Autodesk Inventor part; units mm, degrees
ref_plane "Work Plane2" through (0, 0, 2.5) normal (0, 0, 1) x (1, 0, 0)
ref_plane "Work Plane8" through (0, 0, 0) normal (0.9396926, 0.3420201, 0) x (0, 0, 1)
ref_plane "Work Plane9" through (0, 0, 0) normal (1, 0, 0) x (0, 1, 0)
sketch "Sketch1" plane through (0, 0, 0) normal (0, 0, 1) x (1, 0, 0)
  circle A0 centre (0, 0) radius 16.4903
  dimension "d0" = 32.9806
extrude "Extrusion1" add sketch "Sketch1" along normal blind 5
ref_plane "Work Plane2" through (0, 0, 2.5) normal (0, 0, 1) x (1, 0, 0)
sketch "Sketch2" plane through (0, 0, 0) normal (0, 0, -1) x (-1, 0, 0)
  circle A0 centre (0, 0) radius 16.4903
  circle A1 centre (0, 0) radius 13.5855
  dimension "d3" = 27.171
surface extrude "Pitch Diameter" sketch "Sketch2" against normal through all shown no curves A1
ref_plane "Work Plane8" through (0, 0, 0) normal (0.9396926, 0.3420201, 0) x (0, 0, 1)
ref_plane "Work Plane9" through (0, 0, 0) normal (1, 0, 0) x (0, 1, 0)
spur gear teeth "Spur Gear" teeth 9 pitch diameter 27 tip diameter 32.9806 root diameter 19.5 face width 5 start plane through (0, 0, 0) normal (0, 0, -1) x (-1, 0, 0)
sketch "Sketch3" plane through (0, 0, 5) normal (0, 0, 1) x (1, 0, 0)
  circle A0 centre (0, 0) radius 7.5
  line L0 (0, 0) -> (0, 5)
  line L1 (0, 5) -> (-5.5902, 5)
  line L2 (0, 5) -> (5.5902, 5)
  line L3 (0, 0) -> (0, -5)
  line L4 (0, -5) -> (5.5902, -5)
  line L5 (0, -5) -> (-5.5902, -5)
  dimension "d49" = 15
  dimension "d50" = 5
  dimension "d51" = 5
extrude "Extrusion2" add sketch "Sketch3" along normal blind 40 contours A0 L4 L3 L0 L2 | L1 L0 L3 L5 A0
equation "\"d0\" = da_da"
equation "\"d1\" = da_b"
equation "\"d3\" = da_dw"
equation "\"d16\" = da_aw"
equation "\"d43\" = da_aw"
equation "\"d46\" = da_aw"
properties part number "Drive_Spur" material "Steel"
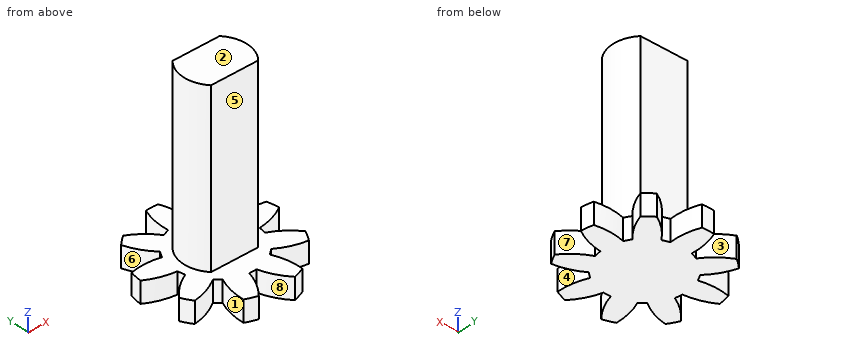
Build history of the part. All positions in model axes, mm. Face numbers are marked on the shaded views. A direction names the side the tool comes from. Round coordinates to 2 decimals unless told otherwise and drop trailing zeros. Write each loop counter-clockwise with the first axis right and the second up, starting at its lowest first coordinate (ties: lowest second). Pieces come first, ordered by that corner, then holes. Notation, with made-up numbers: M 19,53.25 L 28,53.25 A24 cw 28,88.25 Z; hole C 30,-28.5 d2. An arc over 180 degrees is marked long. Answer in a Markdown table with one row per item.
1. Saw through at B-B (x = -11). List the corners of the cut face in (y, z), and give its area (3 significant figures).
Geometry check:
| item | result |
|---|---|
| outline | M -8.9,0 L -3.39,0 L -3.39,5 L -8.9,5 Z; M -0.67,0 L 4.52,0 L 4.52,5 L -0.67,5 Z; M 9.96,0 L 12.29,0 L 12.29,5 L 9.96,5 Z |
| area | 65.2 mm2 |
2. Which spindle directions (+Z, -Z, +X, -X, +Y, -Y) get a long thin tool onto all of the face, cutting with end or side? Do the marked faces 4, 5, 6, 7 and 8. Say none if no direction does.
Geometry check:
| item | result |
|---|---|
| face 4 | +Z, -Z |
| face 5 | +Z, +X, -X, -Y |
| face 6 | +Z, -Z, -X |
| face 7 | +Z, -Z, +X |
| face 8 | +Z, -Z, -Y |
3. Saw through at C-C (y = -6). List the corners of the cut face in (x, z).
Geometry check:
| item | result |
|---|---|
| outline | M -14.13,0 L 14.13,0 L 14.13,5 L -14.13,5 Z |
4. Probe L1, parallel to Z at x = 13.5, y = 3.5; L2, parallel to Y at x = -0.5, z = 38; L3, parallel to X at y = 1.5, z = 11. List the from-to ranges inside material, lowest first. Write a range as [from, to].
Geometry check:
| item | result |
|---|---|
| L1 | [0, 5] |
| L2 | [-5, 5] |
| L3 | [-7.35, 7.35] |
5. Saw through at A-A (x = 12.5). List the corners of the cut face in (y, z), and give its area (3 significant figures).
Geometry check:
| item | result |
|---|---|
| outline | M -9.29,0 L -4.47,0 L -4.47,5 L -9.29,5 Z; M -0.32,0 L 4.61,0 L 4.61,5 L -0.32,5 Z |
| area | 48.8 mm2 |
6. Saw through at D-D (z = 31.5). List the corners of the cut face in (x, y).
Geometry check:
| item | result |
|---|---|
| outline | M -5.59,-5 L 5.59,-5 A7.5 ccw 5.59,5 L -5.59,5 A7.5 ccw Z |
7. Mould opens along Y. For the marked faces 1, 2 and 3 say: +Y half, -Y half, draft (parallel to the pull), parting line (faces both ways), or undercut.
Geometry check:
| item | result |
|---|---|
| face 1 | undercut |
| face 2 | draft |
| face 3 | +Y half |
8. Flat gauge pins, fed straight in: P1, Ø6, axis at x = -11.5, z = 26.5, coming from the -Y side; P2, Ø1, axis at y = 0.5, z = 17.5, coming from the -X side; P3, Ø1, axis at x = 2.5, z = 24, coming from the -Y side; P4, Ø2, axis at y = 1.5, z = 14.5, coming from the +X side. Where does each tip first touch, or does it go through?
Geometry check:
| item | result |
|---|---|
| P1 | through |
| P2 | x = -7.5 |
| P3 | y = -5 |
| P4 | x = 7.48 |
